Input: part model. Units: mm. Frame: model coordinates. A direction names the side the tool comes from. Coordinates: 2 decimals unless noted, no trailing zeros. Loops run counter-clockwise (first coordinate to the right, second up) from the corner with the lowest first, then second, coordinate; pieces in that order, holes last. Notation, with made-up numbers: M -4.5,61.25 L 7.5,61.25 A9 ccw 7.5,75.25 Z; hole C 82.25,41.5 d10. An arc over 180 degrees is marked long. Use a Markdown table: item, result. Add a question column.
1. Section A-A on x = 0. Output: boundary loops of the cut face in (y, z), then the cut area to 3 significant figures.
2. Line query: L1, parallel to Y at x = 3.5, z = 2.75; L2, parallel to X at y = 20, z = 0.25; L3, parallel to Y at x = -2, z = -1. Output: solid intervals per line, ascending. Write a range as [from, to].
3. Section B-B on y = 48. Output: boundary loops of the cut face in (x, z).
4. Pin query (flat end, axial travel): pin 1 (1 mm diameter, centred on x = -2, y = 57, fed in from +Z); pin 2 (1.5 mm diameter, centred on y = 31, z = 1, fed in from +X); pin 3 (6 mm diameter, centred on y = 9.5, z = -4, fed in from +X). Return the tip coordinate at first contact, or that it passes through.
5. Draft query along X for faces 3 (the cylindrical face through (5.037, 34.196, -0.661)), 4 (the flat face through (-2, 68.58, 2)), 5 (the flat face through (2.19, 66.08, 1.29)). Return one class per face: +X half, -X half, draft (parallel to the pull), parting line (faces both ways), or undercut.
6. Set-up query: faces 1 (the flat face through (0, 0, 0)), 2 (the flat face through (2.21, 66.08, -1.25)). Return all of +Z, -Z, +X, -X, +Y, -Y with unobstructed straight access to the full face (end or side cutting, diameter ignored); none if empty.
```python
from build123d import *

# Parameters (mm, degrees)
SKETCH1_R           = 5.08
BOSS_EXTRUDE1_DEPTH = 68.58
CUT_EXTRUDE1_DEPTH  = 5.08
FILLET1_R           = 0.762


with BuildPart() as part:
    # Sketch1 → Boss-Extrude1 (new body)
    with BuildSketch(Plane(origin=(0, 0, 0), x_dir=(1, 0, 0), z_dir=(0, 1, 0))):
        with Locations(Location((0, 0, 0), (0, 0, 270))):
            Circle(SKETCH1_R)
    extrude(amount=BOSS_EXTRUDE1_DEPTH)

    # Sketch2 → Cut-Extrude1 (cut)
    with BuildSketch(Plane(origin=(0, 68.58, 0), x_dir=(1, 0, 0), z_dir=(0, 1, 0))):
        Polygon((-1.466469684, -2.54), (1.466469684, -2.54), (2.932939367, 0), (1.466469684, 2.54), (-1.466469684, 2.54), (-2.932939367, 0), align=None)
    extrude(amount=-CUT_EXTRUDE1_DEPTH, mode=Mode.SUBTRACT)

    # Fillet1
    fillet1_edges = [part.edges().sort_by_distance(p)[0] for p in [
        (0, 0, -5.08),
    ]]
    fillet(fillet1_edges, radius=FILLET1_R)


solid = part.part
```
Answers below:
| question | item | result |
|---|---|---|
| 1 | outline | M 0,-4.32 A0.76 ccw 0.76,-5.08 L 68.58,-5.08 L 68.58,-2.54 L 63.5,-2.54 L 63.5,2.54 L 68.58,2.54 L 68.58,5.08 L 0.76,5.08 A0.76 ccw 0,4.32 Z |
| 1 | area | 671 mm² |
| 2 | L1 | y = [0.01, 68.58] |
| 2 | L2 | x = [-5.07, 5.07] |
| 2 | L3 | y = [0, 63.5] |
| 3 | outline | C 0,0 d10.16 |
| 4 | pin 1 | stops at z = 4.85 |
| 4 | pin 2 | stops at x = 5.07 |
| 4 | pin 3 | stops at x = 4.98 |
| 5 | face 3 | parting line |
| 5 | face 4 | draft |
| 5 | face 5 | undercut |
| 6 | face 1 | +Z, -Z, +X, -X, -Y |
| 6 | face 2 | +Y |
